```python
from build123d import *

# Parameters (mm, degrees)
SKETCH2_W           = 180
SKETCH2_H           = 80
BOSS_EXTRUDE1_DEPTH = 3.18
SKETCH3_W           = 3.18
SKETCH3_H           = 40.18
CUT_EXTRUDE1_DEPTH  = 3.18
SKETCH4_W           = 90.18
SKETCH4_H           = 3.12
CUT_EXTRUDE2_DEPTH  = 3.18
SKETCH5_W           = 3.18
SKETCH5_H           = 19.91
CUT_EXTRUDE3_DEPTH  = 3.18
SKETCH7_R           = 1.5
CUT_EXTRUDE4_DEPTH  = 3.18
SKETCH9_W           = 15
SKETCH9_H           = 3.18
CUT_EXTRUDE6_DEPTH  = 4.18


with BuildPart() as part:
    # Sketch2 → Boss-Extrude1 (new body)
    with BuildSketch(Plane(origin=(0, 0, 0), x_dir=(0, 0, -1), z_dir=(1, 0, 0))):
        Rectangle(SKETCH2_W, SKETCH2_H)
    extrude(amount=BOSS_EXTRUDE1_DEPTH)

    # Sketch3 → Cut-Extrude1 (cut)
    with BuildSketch(Plane(origin=(3.18, 0, 0), x_dir=(0, 0, -1), z_dir=(1, 0, 0))):
        with Locations((-88.41, 0)):
            Rectangle(SKETCH3_W, SKETCH3_H)
    extrude(amount=-CUT_EXTRUDE1_DEPTH, mode=Mode.SUBTRACT)

    # Sketch4 → Cut-Extrude2 (cut)
    with BuildSketch(Plane(origin=(3.18, 0, 0), x_dir=(0, 0, -1), z_dir=(1, 0, 0))):
        with Locations((0, 38.44)):
            Rectangle(SKETCH4_W, SKETCH4_H)
    cut_extrude2 = extrude(amount=-CUT_EXTRUDE2_DEPTH, mode=Mode.SUBTRACT)

    # Mirror1: Cut-Extrude2 across plane
    add(cut_extrude2.mirror(Plane.ZX), mode=Mode.SUBTRACT)

    # Sketch5 → Cut-Extrude3 (cut)
    with BuildSketch(Plane(origin=(3.18, 0, 0), x_dir=(0, 0, -1), z_dir=(1, 0, 0))):
        with Locations((88.41, 30.045)):
            Rectangle(SKETCH5_W, SKETCH5_H)
    cut_extrude3 = extrude(amount=-CUT_EXTRUDE3_DEPTH, mode=Mode.SUBTRACT)

    # Mirror2: Cut-Extrude3 across plane
    add(cut_extrude3.mirror(Plane.ZX), mode=Mode.SUBTRACT)

    # Sketch7 → Cut-Extrude4 (cut)
    with BuildSketch(Plane(origin=(3.18, 0, 0), x_dir=(0, 0, -1), z_dir=(1, 0, 0))):
        with Locations((64.82, 30)):
            Circle(SKETCH7_R)
        with Locations((14.02, 14.7)):
            Circle(SKETCH7_R)
        with Locations((14.02, -13.2)):
            Circle(SKETCH7_R)
        with Locations((66.32, -18.3)):
            Circle(SKETCH7_R)
    extrude(amount=-CUT_EXTRUDE4_DEPTH, mode=Mode.SUBTRACT)

    # Sketch9 → Cut-Extrude6 (cut, through all)
    with BuildSketch(Plane.ZY):
        with Locations((55, -18.41)):
            Rectangle(SKETCH9_W, SKETCH9_H)
    extrude(amount=-CUT_EXTRUDE6_DEPTH, mode=Mode.SUBTRACT)


solid = part.part
```
Input: part model. Units: mm. Frame: model coordinates. A direction names the side the tool comes from. Round coordinates to 2 decimals unless told otherwise and drop trailing zeros. Loops run counter-clockwise (first coordinate to the right, second up) from the corner with the lowest first, then second, coordinate; pieces in that order, holes last. Notation, with made-up numbers: (11, -8.5) -> (61, -8.5) arc R22 cw to (61, -2.5) -> close; hole circle Ø4 at (3.25, 78.25). An arc over 180 degrees is marked (long way). Use one line per item in the form item = value. Start each with the question number.
Item 1: Contact query for flat-ended pins moving along their axis: pin 1 Ø3.5 at (y, z) = (-13.2, -14.02) entering from +X; pin 2 Ø1 at (x, z) = (0.5, -27.5) entering from -Y; pin 3 Ø1.6 at (x, y) = (1.5, -26) entering from -Z; pin 4 Ø1 at (x, y) = (1.5, 12) entering from +Z. Output: stop coordinate, or through.
Item 2: Material intervals for L1, parallel to Y at x = 0.9, z = -14.02; L2, parallel to Y at x = 2.4, z = 58; L3, parallel to Z at x = 0.6, y = -4, sorted ascending. Write a range as from..to.
Item 3: Section query A-A on x = 1.9. Return the cut outline in (y, z).
Item 4: Section query B-B on y = -7. Return the cut outline in (x, z), then the cut area to 3 significant figures.
Item 5: Mould query, pull axis Z, two halves, no side actions, for faces 1 (the face through (2, 30, 90)), 2 (the face through (1.6, 31, -63.7)), 3 (the face through (2, -40, 68)). Classes: pulls with the +Z half, pulls with the -Z half, needs draft (parallel to the pull), parting line crosses it, or undercut.
Item 6: Set-up query: faces 4 (the face through (2, -38, -45.09)), 5 (the face through (2, 0, 86.82)), 6 (the face through (2, 20.09, -88)), 7 (the face through (2, -18, 47.5)). Return all of +Z, -Z, +X, -X, +Y, -Y with unobstructed straight access to the full face (end or side cutting, diameter ignored); none if empty.
Ans:
q1.pin_1 = 3.18
q1.pin_2 = -36.88
q1.pin_3 = -86.82
q1.pin_4 = 86.82
q2.L1 = -36.88..-14.7, -11.7..13.2, 16.2..36.88
q2.L2 = -40..-20, -16.82..40
q2.L3 = -90..86.82
q3.outline = (-40, -86.82) -> (-20.09, -86.82) -> (-20.09, -90) -> (20.09, -90) -> (20.09, -86.82) -> (40, -86.82) -> (40, -45.09) -> (36.88, -45.09) -> (36.88, 45.09) -> (40, 45.09) -> (40, 90) -> (20.09, 90) -> (20.09, 86.82) -> (-20.09, 86.82) -> (-20.09, 90) -> (-40, 90) -> (-40, 45.09) -> (-36.88, 45.09) -> (-36.88, -45.09) -> (-40, -45.09) -> close; hole (-20, 47.5) -> (-16.82, 47.5) -> (-16.82, 62.5) -> (-20, 62.5) -> close; hole circle Ø3 at (-18.3, -66.32); hole circle Ø3 at (-13.2, -14.02); hole circle Ø3 at (14.7, -14.02); hole circle Ø3 at (30, -64.82)
q4.outline = (0, -90) -> (3.18, -90) -> (3.18, 86.82) -> (0, 86.82) -> close
q4.area = 562 mm^2
q5.face_1 = pulls with the +Z half
q5.face_2 = undercut
q5.face_3 = needs draft
q6.face_4 = +X, -X, -Y
q6.face_5 = +Z, +X, -X
q6.face_6 = -Z, +X, -X, +Y
q6.face_7 = +X, -X
